CAD build for the part. Positions are in the model's coordinates, mm. Coordinates: 2 decimals unless noted, no trailing zeros. Order: outer loops, then holes, each group sorted by start corner. A loop starts at its lowest first (then second) coordinate and runs counter-clockwise, first axis right, second up. Notation, with made-up numbers: M -28.5,43.5 L 12.5,43.5 A19 cw 12.5,55.5 Z; hole C 24,-18 d1. An arc over 180 degrees is marked long. One line per item, written item: value.
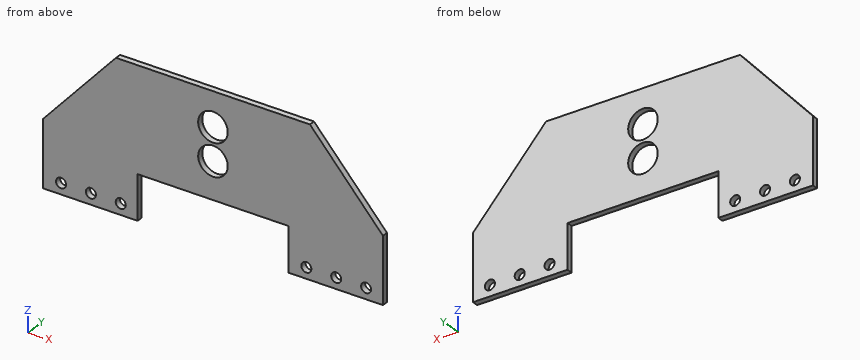
from build123d import *

# Parameters (mm, degrees)
F0_R     = 2.159
F0_R_2   = 6.35
F1_DEPTH = 2.54


with BuildPart() as f1:
    # F0 (on Front) → F1 (new body)
    with BuildSketch(Plane.XZ):
        Polygon((73.025, -3.429), (41.656, 31.75), (32.385, 31.75), (-32.385, 31.75), (-41.656, 31.75), (-73.025, -3.429), (-73.025, -12.7), (-73.025, -31.75), (-32.385, -31.75), (-32.385, -12.7), (32.385, -12.7), (32.385, -31.75), (73.025, -31.75), (73.025, -12.7), align=None)
        with Locations((-65.278, -27.051)):
            Circle(F0_R, mode=Mode.SUBTRACT)
        with Locations((-52.451, -27.051)):
            Circle(F0_R, mode=Mode.SUBTRACT)
        with Locations((-39.624, -27.051)):
            Circle(F0_R, mode=Mode.SUBTRACT)
        with Locations((40.132, -27.051)):
            Circle(F0_R, mode=Mode.SUBTRACT)
        with Locations((52.959, -27.051)):
            Circle(F0_R, mode=Mode.SUBTRACT)
        with Locations((65.786, -27.051)):
            Circle(F0_R, mode=Mode.SUBTRACT)
        with Locations((0, 3.175)):
            Circle(F0_R_2, mode=Mode.SUBTRACT)
        with Locations((0, 17.0688)):
            Circle(F0_R_2, mode=Mode.SUBTRACT)
    extrude(amount=F1_DEPTH)


solid = f1.part
Q1. Slice it at D-D (z = 6.5). List the corners of the cut face in (x, y).
Recorded:
outline: M -64.17,-2.54 L -5.41,-2.54 L -5.41,0 L -64.17,0 Z; M 5.41,-2.54 L 64.17,-2.54 L 64.17,0 L 5.41,0 Z
Q2. Slice it at C-C (y = -0.5). Give the number of separate pieces and of enclosed holes in the cut face, plus the area to 3 significant figures.
Recorded:
separate pieces: 1
enclosed holes: 8
area: 6,600 mm^2
Q3. Slice it at A-A (x = 0). List the corners of the cut face in (y, z) (3 decimals).
Recorded:
outline: M -2.54,-12.7 L 0,-12.7 L 0,-3.175 L -2.54,-3.175 Z; M -2.54,9.525 L 0,9.525 L 0,10.719 L -2.54,10.719 Z; M -2.54,23.419 L 0,23.419 L 0,31.75 L -2.54,31.75 Z
Q4. Pin check, flat tip, straight feed: pin 1 Ø3.5 at (x, z) = (-65.278, -27.051) entering from -Y. Stop position of the tip, or through.
Recorded:
pin 1: passes through
Q5. Drill centre lines: line 1 along X through (y, z) = (-1.5, -20.5) (3 decimals); line 2 along Z through (x, y) = (0, -1.55) (3 decimals); line 3 along Z through (x, y) = (-3.5, -1.25). Where is each one in solid material? Low to high.
Recorded:
line 1: x = -73.025 to -32.385, 32.385 to 73.025
line 2: z = -12.7 to -3.175, 9.525 to 10.719, 23.419 to 31.75
line 3: z = -12.7 to -2.12, 8.47 to 11.77, 22.37 to 31.75
Q6. Slice it at B-B (z = -0.5). List the corners of the cut face in (x, y), plus the area to 3 significant figures.
Recorded:
outline: M -70.41,-2.54 L -5.18,-2.54 L -5.18,0 L -70.41,0 Z; M 5.18,-2.54 L 70.41,-2.54 L 70.41,0 L 5.18,0 Z
area: 331 mm^2
